Autodesk Inventor part; units mm, degrees
ref_plane "YZ Plane" through (0, 0, 0) normal (1, 0, 0) x (0, 1, 0)
ref_plane "XZ Plane" through (0, 0, 0) normal (0, 1, 0) x (-1, 0, 0)
ref_plane "XY Plane" through (0, 0, 0) normal (0, 0, 1) x (1, 0, 0)
sketch "Sketch1" plane through (0, 0, 0) normal (0, 1, 0) x (-1, 0, 0)
  line L0 (-74.6125, -18.1483) -> (74.6125, -18.1483)
  line L1 (74.6125, -18.1483) -> (74.6125, 18.1483)
  line L2 (74.6125, 18.1483) -> (-74.6125, 18.1483)
  line L3 (-74.6125, 18.1483) -> (-74.6125, -18.1483)
  line L4 (74.6125, -18.1483) -> (37.8079, -18.1483)
  line L5 (37.8079, -18.1483) -> (37.8079, 18.1483)
  line L6 (37.8079, 18.1483) -> (74.6125, 18.1483)
  line L7 (74.6125, 18.1483) -> (74.6125, -18.1483)
  line L8 (21.7678, 18.1483) -> (-74.6125, 18.1483)
  line L9 (-74.6125, 18.1483) -> (-74.6125, -18.1483)
  line L10 (-74.6125, -18.1483) -> (21.7678, -18.1483)
  line L11 (21.7678, -18.1483) -> (21.7678, 18.1483)
  line L12 (59.5566, 2.667) -> (42.1449, 2.667)
  line L13 (42.1449, 2.667) -> (42.1449, -2.667)
  line L14 (42.1449, -2.667) -> (59.5566, -2.667)
  line L15 (59.5566, -2.667) -> (59.5566, 2.667)
  line L16 (53.5178, 8.7058) -> (48.1838, 8.7058)
  line L17 (48.1838, 8.7058) -> (48.1838, -8.7058)
  line L18 (48.1838, -8.7058) -> (53.5178, -8.7058)
  line L19 (53.5178, -8.7058) -> (53.5178, 8.7058)
  circle A0 centre (-47.8282, 0) radius 3.7846
  circle A1 centre (-35.1917, 0) radius 3.7846
  circle A2 centre (28.2448, 0) radius 5.4546
  point P0 (0, 0)
  point P1 (50.8508, 0)
  dimension "d0" = 149.225
  dimension "d1" = 36.2966
  dimension "d2" = 36.8046
  dimension "d11" = 17.4117
  dimension "d12" = 5.334
  dimension "d13" = 5.334
  dimension "d14" = 17.4117
  dimension "d15" = 7.5692
  dimension "d16" = 7.5692
  dimension "d17" = 10.9093
extrude "Battery" add sketch "Sketch1" against normal blind 31.2166 contours L3 L2 L11 L0 | A0 | A1
extrude "Sensor" add sketch "Sketch1" against normal blind 20.7391 contours L5 L2 L1 L0 | L15 L14 L19 L12 | L19 L14 L17 L12 | L12 L17 L16 L19 | L17 L14 L13 L12 | L19 L18 L17 L14
loft "Loft1" add section 1 edges at (-37.8079, 0, 0) (-37.8079, -10.3696, 18.1483) (-37.8079, -20.7391, 0) (-37.8079, -10.3696, -18.1483) section 2 edges at (-21.7678, 0, 0) (-21.7678, -15.6083, -18.1483) (-21.7678, -31.2166, 0) (-21.7678, -15.6083, 18.1483)
extrude "1 Button" add sketch "Sketch1" along normal blind 2.032 contours A1
extrude "2 Button" add sketch "Sketch1" along normal blind 2.032 contours A0
extrude "A Button" add sketch "Sketch1" along normal blind 2.032 contours A2
extrude "D-Pad" add sketch "Sketch1" along normal blind 2.032 contours L15 L14 L19 L12 | L19 L14 L17 L12 | L12 L17 L16 L19 | L17 L14 L13 L12 | L19 L18 L17 L14
sketch "Sketch2" plane through (0, 0, 0) normal (0, 1, 0) x (1, 0, 0)
  line L0 (57.8104, -18.1483) -> (57.8104, 18.1483)
  line L1 (-64.8843, -18.1483) -> (-64.8843, 18.1483)
  point P0 (0, 0)
properties part number "wiimote"
For this review, take the finished solid that the model builds, in its own axes (mm). A direction names the side the tool comes from. Coordinates: 2 decimals unless noted, no trailing zeros. Loops run counter-clockwise (first coordinate to the right, second up) from the corner with the lowest first, then second, coordinate; pieces in that order, holes last. Notation, with made-up numbers: (27, 8) - (44, 8) arc R37 ccw to (44, 46) - close; hole circle Ø2 at (70.5, 48). An arc over 180 degrees is marked (long way). Use a Markdown table: item, result. Add a question column.
Item 1: Mouldability with a two-part tool opening along X and no side actions: class faces 4 (the face through (31.582, 1.002, -1.137)), 5 (the face through (-29.68, -26.05, 0.25)), 6 (the face through (2, -16, -18.148)) as pulls with the +X half, pulls with the -X half, needs draft (parallel to the pull), parting line crosses it, or undercut.
Item 2: We need section B-B (x = 40.5). Give the boundary of the cut face in (y, z), and give its area (3 significant figures).
Item 3: For line 1 (Y direction, x = 4, z = 10); line 2 (Y direction, x = -41, z = -15); line 3 (X direction, y = -23, z = -12.5), list the stretches that pass through material, from the lowest coordinate up.
Item 4: Insertion check: pin 1 Ø1 at (x, y) = (-51.5, 1) entering from +Z; pin 2 Ø0.6 at (y, z) = (1.5, 4) entering from -X; pin 3 Ø10 at (x, z) = (-14, 6) entering from +Y. Each pin has a flat end and moves straight along its axis. Give the tip position at first contact, or say it passes through.
Item 5: We need section A-A (z = 0). Give the boundary of the cut face in (x, y), and give its area (3 significant figures).
Item 6: Tool access review of faces 1 (the face through (44.332, 1.002, 1.45)), 2 (the face through (-56, -20.739, 0)), 3 (the face through (2, -15, 18.148)): name each direction out of +Z, -Z, +X, -X, +Y, -Y from which nothing blocks a thin tool from reaching the whole face with its end or side.
Item 7: We need section C-C (z = -14.5). Give the boundary of the cut face in (x, y), and give its area (3 significant figures).
Item 8: We need section D-D (x = -28.5). Give the boundary of the cut face in (y, z).
Results list:
| question | item | result |
|---|---|---|
| 1 | face 4 | undercut |
| 1 | face 5 | pulls with the -X half |
| 1 | face 6 | needs draft |
| 2 | outline | (-31.22, -18.15) - (0, -18.15) - (0, 18.15) - (-31.22, 18.15) - close |
| 2 | area | 1,130 mm^2 |
| 3 | line 1 | y = -31.22 to 0 |
| 3 | line 2 | y = -20.74 to 0 |
| 3 | line 3 | x = -34.35 to 74.61 |
| 4 | pin 1 | stops at z = 8.71 |
| 4 | pin 2 | stops at x = -53.52 |
| 4 | pin 3 | stops at y = 0 |
| 5 | outline | (-74.61, -20.74) - (-37.81, -20.74) - (-21.77, -31.22) - (74.61, -31.22) - (74.61, 0) - (51.61, 0) - (51.61, 2.03) - (44.04, 2.03) - (44.04, 0) - (38.98, 0) - (38.98, 2.03) - (31.41, 2.03) - (31.41, 0) - (-22.79, 0) - (-22.79, 2.03) - (-33.7, 2.03) - (-33.7, 0) - (-42.14, 0) - (-42.14, 2.03) - (-59.56, 2.03) - (-59.56, 0) - (-74.61, 0) - close |
| 5 | area | 4,280 mm^2 |
| 6 | face 1 | +Y |
| 6 | face 2 | +Z, -Z, -X, -Y |
| 6 | face 3 | +Z, +X, -X, +Y, -Y |
| 7 | outline | (-74.61, -20.74) - (-37.81, -20.74) - (-21.77, -31.22) - (74.61, -31.22) - (74.61, 0) - (-74.61, 0) - close |
| 7 | area | 4,190 mm^2 |
| 8 | outline | (-26.82, -18.15) - (0, -18.15) - (0, -5.45) - (2.03, -5.45) - (2.03, 5.45) - (0, 5.45) - (0, 18.15) - (-26.82, 18.15) - close |
